For this review, take the finished solid that the model builds, in its own axes (mm). A direction names the side the tool comes from. Coordinates: 2 decimals unless noted, no trailing zeros. Loops run counter-clockwise (first coordinate to the right, second up) from the corner with the lowest first, then second, coordinate; pieces in that order, holes last. Notation, with made-up numbers: (-13, 54) - (19, 54) arc R32 cw to (19, 82) - close; hole circle Ø1 at (-2.5, -14.75). An arc over 180 degrees is marked (long way). Use one line per item in the form item = value. Start each with the question number.
1. For pin 1 Ø1 at (x, z) = (1, 2) entering from +Y; pin 2 Ø0.9 at (y, z) = (0, 2) entering from +X; pin 3 Ø0.5 at (y, z) = (0, 7) entering from +X; pin 4 Ø1.5 at (x, z) = (-1, 7.5) entering from -Y, all flat-tipped, find the tip position at first contact; note any pin that passes through.
2. Add section A-A on z = 2.5. Give the boundary of the cut face in (x, y), and give its area (4 significant figures).
3. Machinability: for faces 1 (the face through (0.955, 0.856, 2.232)), 2 (the face through (-1, 0, 1)), 3 (the face through (1.1, -0.32, 0.4)), 4 (the face through (1.25, 0, 2)), 5 (the face through (1.1, 0.32, 0.4)), which of the approach directions +Z, -Z, +X, -X, +Y, -Y give a long, thin tool a straight path to every point of the face, cutting with its end or side? Answer none if there is none.
4. Add section D-D on x = 1.8. Give the boundary of the cut face in (y, z).
5. Add section B-B on x = 1.1. Give the boundary of the cut face in (y, z), and give its area (3 significant figures).
6. To check wall thickness, follow probe 1 along Z at (x, y) = (0.75, 0.55); probe 2 along X at (y, z) = (0.1, 8.5); probe 3 along Z at (x, y) = (1.45, -0.1). State the ranges of each line that lie inside material, in increasing order.
7. Add section C-C on y = 0.65. Give the boundary of the cut face in (x, z).
```python
from build123d import *
from OCP.BRepFilletAPI import BRepFilletAPI_MakeChamfer

# Parameters (mm, degrees)
SKETCH_1_W           = 2.5
SKETCH_1_H           = 2.5
EXTRUDE_1_DEPTH      = 2.5
EXTRUDE_2_DEPTH      = 6
EXTRUDE_2_DEPTH_BACK = 3.5
SKETCH_2_W           = 0.64
SKETCH_2_H           = 0.64
SKETCH_4_W           = 0.64
SKETCH_4_H           = 0.64
EXTRUDE_4_DEPTH      = 2.5
FILLET_1_R           = 0.5
CHAMFER_1_SIZE       = 0.2
CHAMFER_1_SIZE2      = 0.145308506
CHAMFER_2_SIZE       = 0.8
CHAMFER_2_SIZE2      = 0.581234022


with BuildPart() as part:
    # Эскиз1 → Бобышка-Вытянуть1 (new body)
    with BuildSketch(Plane.XY.offset(1)):
        Rectangle(SKETCH_1_W, SKETCH_1_H)
    extrude(amount=EXTRUDE_1_DEPTH)

    # Эскиз2 → Бобышка-Вытянуть2 (add, two sides: drawn at the far end of the back side and taken through both)
    with BuildSketch(Plane.XY.offset(3.5).offset(-EXTRUDE_2_DEPTH_BACK)):
        Rectangle(SKETCH_2_W, SKETCH_2_H)
    extrude(amount=EXTRUDE_2_DEPTH + EXTRUDE_2_DEPTH_BACK)

    # Эскиз4 → Бобышка-Вытянуть4 (add)
    with BuildSketch(Plane(origin=(0.32, 0, 0), x_dir=(0, 0, -1), z_dir=(1, 0, 0))):
        with Locations((-0.32, 0)):
            Rectangle(SKETCH_4_W, SKETCH_4_H)
    extrude(amount=EXTRUDE_4_DEPTH)

    # Скругление1
    fillet_1_edges = [part.edges().sort_by_distance(p)[0] for p in [
        (-0.32, 0, 0),
    ]]
    fillet(fillet_1_edges, radius=FILLET_1_R)

    # Фаска1: one chamfer whose edges measure the first distance from different faces: ONE call of the kernel's chamfer builder (chamfer() names one face for all edges)
    chamfer_1_edges_1 = [part.edges().sort_by_distance(p)[0] for p in [
        (0.32, 0, 9.5),
    ]]
    chamfer_1_side_1 = [part.faces().sort_by_distance(p)[0] for p in [
        (0.32, 0, 6.5),
    ]]
    chamfer_1_edges_2 = [part.edges().sort_by_distance(p)[0] for p in [
        (0, 0.32, 9.5),
    ]]
    chamfer_1_side_2 = [part.faces().sort_by_distance(p)[0] for p in [
        (0, 0.32, 6.5),
    ]]
    chamfer_1_edges_3 = [part.edges().sort_by_distance(p)[0] for p in [
        (-0.32, 0, 9.5),
    ]]
    chamfer_1_side_3 = [part.faces().sort_by_distance(p)[0] for p in [
        (-0.32, 0, 6.5),
    ]]
    chamfer_1_edges_4 = [part.edges().sort_by_distance(p)[0] for p in [
        (0, -0.32, 9.5),
    ]]
    chamfer_1_side_4 = [part.faces().sort_by_distance(p)[0] for p in [
        (0, -0.32, 6.5),
    ]]
    chamfer_1_edges_5 = [part.edges().sort_by_distance(p)[0] for p in [
        (2.82, 0, 0),
    ]]
    chamfer_1_side_5 = [part.faces().sort_by_distance(p)[0] for p in [
        (1.5, 0, 0),
    ]]
    chamfer_1_edges_6 = [part.edges().sort_by_distance(p)[0] for p in [
        (2.82, 0.32, 0.32),
    ]]
    chamfer_1_side_6 = [part.faces().sort_by_distance(p)[0] for p in [
        (1.154058948, 0.32, 0.3778024),
    ]]
    chamfer_1_edges_7 = [part.edges().sort_by_distance(p)[0] for p in [
        (2.82, 0, 0.64),
    ]]
    chamfer_1_side_7 = [part.faces().sort_by_distance(p)[0] for p in [
        (1.57, 0, 0.64),
    ]]
    chamfer_1_edges_8 = [part.edges().sort_by_distance(p)[0] for p in [
        (2.82, -0.32, 0.32),
    ]]
    chamfer_1_side_8 = [part.faces().sort_by_distance(p)[0] for p in [
        (1.154058948, -0.32, 0.3778024),
    ]]
    chamfer_1 = BRepFilletAPI_MakeChamfer(part.part.solid().wrapped)
    for e in chamfer_1_edges_1:
        chamfer_1.Add(CHAMFER_1_SIZE, CHAMFER_1_SIZE2, e.wrapped, chamfer_1_side_1[0].wrapped)  # the first distance lies on this face
    for e in chamfer_1_edges_2:
        chamfer_1.Add(CHAMFER_1_SIZE, CHAMFER_1_SIZE2, e.wrapped, chamfer_1_side_2[0].wrapped)  # the first distance lies on this face
    for e in chamfer_1_edges_3:
        chamfer_1.Add(CHAMFER_1_SIZE, CHAMFER_1_SIZE2, e.wrapped, chamfer_1_side_3[0].wrapped)  # the first distance lies on this face
    for e in chamfer_1_edges_4:
        chamfer_1.Add(CHAMFER_1_SIZE, CHAMFER_1_SIZE2, e.wrapped, chamfer_1_side_4[0].wrapped)  # the first distance lies on this face
    for e in chamfer_1_edges_5:
        chamfer_1.Add(CHAMFER_1_SIZE, CHAMFER_1_SIZE2, e.wrapped, chamfer_1_side_5[0].wrapped)  # the first distance lies on this face
    for e in chamfer_1_edges_6:
        chamfer_1.Add(CHAMFER_1_SIZE, CHAMFER_1_SIZE2, e.wrapped, chamfer_1_side_6[0].wrapped)  # the first distance lies on this face
    for e in chamfer_1_edges_7:
        chamfer_1.Add(CHAMFER_1_SIZE, CHAMFER_1_SIZE2, e.wrapped, chamfer_1_side_7[0].wrapped)  # the first distance lies on this face
    for e in chamfer_1_edges_8:
        chamfer_1.Add(CHAMFER_1_SIZE, CHAMFER_1_SIZE2, e.wrapped, chamfer_1_side_8[0].wrapped)  # the first distance lies on this face
    add(Compound.cast(chamfer_1.Shape()), mode=Mode.REPLACE)

    # Фаска2: one chamfer whose edges measure the first distance from different faces: ONE call of the kernel's chamfer builder (chamfer() names one face for all edges)
    chamfer_2_edges_1 = [part.edges().sort_by_distance(p)[0] for p in [
        (1.25, -1.25, 2.25),
    ]]
    chamfer_2_side_1 = [part.faces().sort_by_distance(p)[0] for p in [
        (0, -1.25, 2.25),
    ]]
    chamfer_2_edges_2 = [part.edges().sort_by_distance(p)[0] for p in [
        (1.25, 1.25, 2.25),
    ]]
    chamfer_2_side_2 = [part.faces().sort_by_distance(p)[0] for p in [
        (1.25, 0, 2.25),
    ]]
    chamfer_2 = BRepFilletAPI_MakeChamfer(part.part.solid().wrapped)
    for e in chamfer_2_edges_1:
        chamfer_2.Add(CHAMFER_2_SIZE, CHAMFER_2_SIZE2, e.wrapped, chamfer_2_side_1[0].wrapped)  # the first distance lies on this face
    for e in chamfer_2_edges_2:
        chamfer_2.Add(CHAMFER_2_SIZE, CHAMFER_2_SIZE2, e.wrapped, chamfer_2_side_2[0].wrapped)  # the first distance lies on this face
    add(Compound.cast(chamfer_2.Shape()), mode=Mode.REPLACE)


solid = part.part
```
Conclusion:
q1.pin_1 = 1.25
q1.pin_2 = 1.25
q1.pin_3 = 0.32
q1.pin_4 = -0.32
q2.outline = (-1.25, -1.25) - (0.45, -1.25) - (1.25, -0.67) - (1.25, 0.45) - (0.67, 1.25) - (-1.25, 1.25) - close
q2.area = 5.785 mm^2
q3.face_1 = +Z, -Z, +X, +Y
q3.face_2 = none
q3.face_3 = -Z, +X, -X, -Y
q3.face_4 = +Z, +X, +Y, -Y
q3.face_5 = -Z, +X, -X, +Y
q4.outline = (-0.32, 0) - (0.32, 0) - (0.32, 0.64) - (-0.32, 0.64) - close
q5.outline = (-0.78, 1) - (0.66, 1) - (0.66, 3.5) - (-0.78, 3.5) - close; (-0.32, 0) - (0.32, 0) - (0.32, 0.64) - (-0.32, 0.64) - close
q5.area = 4.00 mm^2
q6.probe_1 = 1 to 3.5
q6.probe_2 = -0.32 to 0.32
q6.probe_3 = 0 to 0.64
q7.outline = (-1.25, 1) - (1.1, 1) - (1.1, 3.5) - (-1.25, 3.5) - close
